from build123d import *

# Parameters (mm, degrees)
SKETCH_1_R      = 5
EXTRUDE_1_DEPTH = 4


with BuildPart() as part:
    # Эскиз1 → Бобышка-Вытянуть1 (new body)
    with BuildSketch(Plane.XY):
        with BuildLine():
            Line((8.526879851, 0), (12, 0))
            ThreePointArc((12, 0), (14.121320344, 0.878679656), (15, 3))
            Line((15, 3), (15, 90))
            Line((15, 90), (19, 90))
            ThreePointArc((19, 90), (20.154255418, 88.845744582), (19, 87.691489165))
            Line((19, 87.691489165), (19, 3))
            ThreePointArc((19, 3), (19.878679656, 0.878679656), (22, 0))
            Line((22, 0), (134.07411748, 0))
            ThreePointArc((134.07411748, 0), (165, -14), (195.92588252, 0))
            Line((195.92588252, 0), (304.07411748, 0))
            ThreePointArc((304.07411748, 0), (335, -14), (365.92588252, 0))
            Line((365.92588252, 0), (478, 0))
            ThreePointArc((478, 0), (480.121320344, 0.878679656), (481, 3))
            Line((481, 3), (481, 87.691489165))
            ThreePointArc((481, 87.691489165), (479.845744582, 88.845744582), (481, 90))
            Line((481, 90), (485, 90))
            Line((485, 90), (485, 3))
            ThreePointArc((485, 3), (485.878679656, 0.878679656), (488, 0))
            Line((488, 0), (491.473120149, 0))
            ThreePointArc((491.473120149, 0), (498.004324615, 2.427459592), (501.364682095, 8.531326355))
            ThreePointArc((501.364682095, 8.531326355), (504.376413281, 95.021242555), (488, 180))
            Line((488, 180), (481, 180))
            Line((481, 180), (471, 170))
            Line((471, 170), (454.102752641, 170))
            Line((454.102752641, 170), (444.102752641, 180))
            Line((444.102752641, 180), (425, 180))
            Line((425, 180), (420, 175))
            Line((420, 175), (410, 175))
            Line((410, 175), (405, 180))
            Line((405, 180), (395, 180))
            Line((395, 180), (390, 175))
            Line((390, 175), (380, 175))
            Line((380, 175), (375, 180))
            Line((375, 180), (365, 180))
            Line((365, 180), (360, 175))
            Line((360, 175), (350, 175))
            Line((350, 175), (345, 180))
            Line((345, 180), (335, 180))
            Line((335, 180), (330, 175))
            Line((330, 175), (320, 175))
            Line((320, 175), (315, 180))
            Line((315, 180), (305, 180))
            Line((305, 180), (300, 175))
            Line((300, 175), (290, 175))
            Line((290, 175), (285, 180))
            Line((285, 180), (275, 180))
            Line((275, 180), (270, 175))
            Line((270, 175), (260, 175))
            Line((260, 175), (255, 180))
            Line((255, 180), (245, 180))
            Line((245, 180), (240, 175))
            Line((240, 175), (230, 175))
            Line((230, 175), (225, 180))
            Line((225, 180), (215, 180))
            Line((215, 180), (210, 175))
            Line((210, 175), (200, 175))
            Line((200, 175), (195, 180))
            Line((195, 180), (185, 180))
            Line((185, 180), (180, 175))
            Line((180, 175), (170, 175))
            Line((170, 175), (165, 180))
            Line((165, 180), (155, 180))
            Line((155, 180), (150, 175))
            Line((150, 175), (140, 175))
            Line((140, 175), (135, 180))
            Line((135, 180), (125, 180))
            Line((125, 180), (120, 175))
            Line((120, 175), (110, 175))
            Line((110, 175), (105, 180))
            Line((105, 180), (95, 180))
            Line((95, 180), (90, 175))
            Line((90, 175), (80, 175))
            Line((80, 175), (75, 180))
            Line((75, 180), (55.897247359, 180))
            Line((55.897247359, 180), (45.897247359, 170))
            Line((45.897247359, 170), (29, 170))
            Line((29, 170), (19, 180))
            Line((19, 180), (12, 180))
            ThreePointArc((12, 180), (-4.376413281, 95.021242555), (-1.364682095, 8.531326355))
            ThreePointArc((-1.364682095, 8.531326355), (1.995675385, 2.427459592), (8.526879851, 0))
        make_face()
        with Locations((45.897247359, 70)):
            Circle(SKETCH_1_R, mode=Mode.SUBTRACT)
        with Locations((65.46620575, 45)):
            Circle(SKETCH_1_R, mode=Mode.SUBTRACT)
        with Locations((75, 70)):
            Circle(SKETCH_1_R, mode=Mode.SUBTRACT)
        with Locations((94.568958391, 45)):
            Circle(SKETCH_1_R, mode=Mode.SUBTRACT)
        with Locations((104.102752641, 70)):
            Circle(SKETCH_1_R, mode=Mode.SUBTRACT)
        with Locations((123.671711032, 45)):
            Circle(SKETCH_1_R, mode=Mode.SUBTRACT)
        with Locations((133.205505282, 70)):
            Circle(SKETCH_1_R, mode=Mode.SUBTRACT)
        with Locations((152.774463674, 45)):
            Circle(SKETCH_1_R, mode=Mode.SUBTRACT)
        with Locations((162.308257923, 70)):
            Circle(SKETCH_1_R, mode=Mode.SUBTRACT)
        with Locations((181.877216315, 45)):
            Circle(SKETCH_1_R, mode=Mode.SUBTRACT)
        with Locations((191.411010565, 70)):
            Circle(SKETCH_1_R, mode=Mode.SUBTRACT)
        with Locations((210.979968956, 45)):
            Circle(SKETCH_1_R, mode=Mode.SUBTRACT)
        with Locations((220.513763206, 70)):
            Circle(SKETCH_1_R, mode=Mode.SUBTRACT)
        with Locations((240.082721597, 45)):
            Circle(SKETCH_1_R, mode=Mode.SUBTRACT)
        with Locations((249.616515847, 70)):
            Circle(SKETCH_1_R, mode=Mode.SUBTRACT)
        with Locations((269.185474238, 45)):
            Circle(SKETCH_1_R, mode=Mode.SUBTRACT)
        with Locations((278.719268488, 70)):
            Circle(SKETCH_1_R, mode=Mode.SUBTRACT)
        with Locations((298.288226879, 45)):
            Circle(SKETCH_1_R, mode=Mode.SUBTRACT)
        with Locations((307.822021129, 70)):
            Circle(SKETCH_1_R, mode=Mode.SUBTRACT)
        with Locations((327.39097952, 45)):
            Circle(SKETCH_1_R, mode=Mode.SUBTRACT)
        with Locations((336.92477377, 70)):
            Circle(SKETCH_1_R, mode=Mode.SUBTRACT)
        with Locations((356.493732162, 45)):
            Circle(SKETCH_1_R, mode=Mode.SUBTRACT)
        with Locations((366.027526411, 70)):
            Circle(SKETCH_1_R, mode=Mode.SUBTRACT)
        with Locations((385.596484803, 45)):
            Circle(SKETCH_1_R, mode=Mode.SUBTRACT)
        with Locations((395.130279053, 70)):
            Circle(SKETCH_1_R, mode=Mode.SUBTRACT)
        with Locations((414.699237444, 45)):
            Circle(SKETCH_1_R, mode=Mode.SUBTRACT)
        with Locations((425, 70)):
            Circle(SKETCH_1_R, mode=Mode.SUBTRACT)
        with Locations((444.568958391, 45)):
            Circle(SKETCH_1_R, mode=Mode.SUBTRACT)
        with Locations((454.869720947, 70)):
            Circle(SKETCH_1_R, mode=Mode.SUBTRACT)
        with BuildLine():
            Line((152, 6), (178, 6))
            Line((178, 6), (178, 9))
            ThreePointArc((178, 9), (179.414213562, 12.414213562), (176, 11))
            Line((176, 11), (154, 11))
            ThreePointArc((154, 11), (150.585786438, 12.414213562), (152, 9))
            Line((152, 9), (152, 6))
        make_face(mode=Mode.SUBTRACT)
        with BuildLine():
            Line((322, 6), (348, 6))
            Line((348, 6), (348, 9))
            ThreePointArc((348, 9), (349.414213562, 12.414213562), (346, 11))
            Line((346, 11), (324, 11))
            ThreePointArc((324, 11), (320.585786438, 12.414213562), (322, 9))
            Line((322, 9), (322, 6))
        make_face(mode=Mode.SUBTRACT)
    extrude(amount=EXTRUDE_1_DEPTH)


solid = part.part
Geometry: final body of the model. Coordinates: model frame, mm. A direction names the side the tool comes from. Round coordinates to 2 decimals unless told otherwise and drop trailing zeros. Order: outer loops, then holes, each group sorted by start corner. A loop starts at its lowest first (then second) coordinate and runs counter-clockwise, first axis right, second up.
Q1. Mould query, pull axis X, two halves, no side actions, for faces 1 (the face through (50.666, 71.502, 1.972)), 2 (the face through (497.929, 2.363, 1.972)), 3 (the face through (246, 84, 0)). Classes: released by +X, released by -X, zero draft, split by the parting line, or undercut.
Result sheet:
face 1: undercut
face 2: released by +X
face 3: zero draft
Q2. Pin query (flat end, axial travel): pin 1 (13 mm diameter, centred on x = 133.21, y = 70, fed in from -Z); pin 2 (2 mm diameter, centred on x = 311.5, y = 69, fed in from +Z); pin 3 (2 mm diameter, centred on x = 339, z = 2.5, fed in from -Y); pin 4 (2 mm diameter, centred on x = 234, z = 2.5, fed in from +Y). Return the tip coordinate at first contact, or that it passes through.
Result sheet:
pin 1: stops at z = 0
pin 2: passes through
pin 3: stops at y = -13.89
pin 4: stops at y = 175
Q3. Section A-A, the plane y = 26. Output: boundary loops of the cut face in (x, z), and give its area (3 significant figures).
Result sheet:
outline: (-3.55, 0) - (15, 0) - (15, 4) - (-3.55, 4) - close; (19, 0) - (481, 0) - (481, 4) - (19, 4) - close; (485, 0) - (503.55, 0) - (503.55, 4) - (485, 4) - close
area: 2,000 mm2
Q4. Section C-C, the plane y = 135. Output: boundary loops of the cut face in (x, z).
Result sheet:
outline: (0.86, 0) - (499.14, 0) - (499.14, 4) - (0.86, 4) - close
Q5. Material intervals for probe 1 along Y at (x, z) = (269.5, 0.3); probe 2 along Y at (x, z) = (333.5, 1.15); probe 3 along X at (y, z) = (25.5, 0.5), sorted ascending.
Result sheet:
probe 1: y = 0 to 40.01, 49.99 to 175
probe 2: y = -13.97 to 6, 11 to 66.36, 73.64 to 178.5
probe 3: x = -3.5 to 15, 19 to 481, 485 to 503.5
Q6. Access query for faces 4 (the face through (476, 175, 2)), 5 (the face through (335, -14, 2)). Directions: +Z, -Z, +X, -X, +Y, -Y. A direction counts if a zero-diameter tool reaches every point of the face in a straight line with its end or side. Return the directions, or none.
Result sheet:
face 4: +Z, -Z, +Y
face 5: +Z, -Z, -Y
Q7. Section B-B, the plane z = 0.9. Give the number of separate pieces and of enclosed holes in the cut face, and give its area (3 significant figures).
Result sheet:
separate pieces: 1
enclosed holes: 31
area: 86,800 mm2
